Here's how the part is built. I have some questions about the finished solid (model axes, mm). A direction names the side the tool comes from. Coordinates: 2 decimals unless noted, no trailing zeros. Order: outer loops, then holes, each group sorted by start corner. A loop starts at its lowest first (then second) coordinate and runs counter-clockwise, first axis right, second up. Notation, with made-up numbers: (10.5, 8.25) - (60.5, 8.25) arc R31 cw to (60.5, 42.25) - close; hole circle Ø8 at (-36.75, -28). An arc over 180 degrees is marked (long way). Answer in a Markdown table with one row per item. Add a question column.
Item 1: Thinking about a two-plate mould opening in Z: for faces 1 (the flat face through (3.3, 0.1, -3.4)), 2 (the flat face through (1.03, 1.74, -0.99)), 3 (the cylindrical face through (18, -3, 0)), 4 (the conical face through (3.05, -0.07, -0.31)), which applies, +Z half, -Z half, draft (parallel to the pull), parting line (faces both ways), or undercut?
Item 2: If I drill on line 1 along Z through (x, y) = (26.5, 0); line 2 along Z through (x, y) = (1.5, -1); line 3 along X through (y, z) = (-2.75, -3.25), over which ranges is the centre line in solid material (lowest first)? Write a range as from..to.
Item 3: I want a section at A-A (x = 16). Please give me the cut outline in (y, z), plus the area to 3 significant figures.
Item 4: I want a section at B-B (y = 4.75). Please give me the cut outline in (x, z), plus the area to 3 significant figures.
Item 5: Will these pins go through, and if not, where does the flat tip stop? pin 1 Ø1 at (x, y) = (22.5, -2.5) entering from -Z; pin 2 Ø1.7 at (x, y) = (1, -0.5) entering from +Z; pin 3 Ø4 at (x, y) = (13.5, -2.5) entering from -Z; pin 4 Ø6 at (x, z) = (5, 0) entering from +Y.
Item 6: On a 3-axis mill with a long thin cutter (end or side, diameter ignored), from which of +Z, -Z, +X, -X, +Y, -Y can I reach the whole of each face in a straight line? I mean faces 5 (the flat face through (0, -2, -1)), 6 (the flat face through (1.03, -1.74, 0.99)). Say none if no direction works.
```python
from build123d import *

# Parameters (mm, degrees)
FILLET1_R   = 0.25
HEX_2_DEPTH = 2.08


with BuildPart() as part:
    # BodySke → BaseBody (revolve)
    with BuildSketch(Plane.XY):
        with BuildLine():
            Line((33.3, 0), (33.3, 2.4455))
            Line((33.3, 2.4455), (32.7455, 3))
            Line((32.7455, 3), (3.3, 3))
            Line((3.3, 3), (3.3, 5.25))
            Line((3.3, 5.25), (2.92, 5.25))
            ThreePointArc((2.92, 5.25), (1.224500646, 4.199464996), (0, 2.625))
            Line((0, 2.625), (0, 0))
            Line((0, 0), (33.3, 0))
        make_face()
    revolve(axis=Axis((0, 0, 0), (1, 0, 0)))

    # Fillet1
    fillet1_edges = [part.edges().sort_by_distance(p)[0] for p in [
        (3.3, -3, 0),
    ]]
    fillet(fillet1_edges, radius=FILLET1_R)

    # Sketch2 → PreBroach (revolve, cut)
    with BuildSketch(Plane.XY):
        Polygon((0, 2), (2.08, 2), (3.234700538, 0), (0, 0), align=None)
    revolve(axis=Axis((0, 0, 0), (1, 0, 0)), mode=Mode.SUBTRACT)

    # Sketch3 → Hex 2 (cut)
    with BuildSketch(Plane(origin=(0, 0, 0), x_dir=(0, 0, -1), z_dir=(1, 0, 0))):
        Polygon((-2, -1.154700538), (-2, 1.154700538), (0, 2.309401077), (2, 1.154700538), (2, -1.154700538), (0, -2.309401077), align=None)
    extrude(amount=HEX_2_DEPTH, mode=Mode.SUBTRACT)


solid = part.part
```
Values follow:
| question | item | result |
|---|---|---|
| 1 | face 1 | draft |
| 1 | face 2 | undercut |
| 1 | face 3 | parting line |
| 1 | face 4 | undercut |
| 2 | line 1 | z = -3..3 |
| 2 | line 2 | z = -4.32..-2, 2..4.32 |
| 2 | line 3 | x = 1.29..3.3 |
| 3 | outline | circle Ø6 at (0, 0) |
| 3 | area | 28.3 mm^2 |
| 4 | outline | (2.92, -2.24) - (3.3, -2.24) - (3.3, 2.24) - (2.92, 2.24) arc R3.05 ccw to start |
| 4 | area | 4.71 mm^2 |
| 5 | pin 1 | stops at z = -2.24 |
| 5 | pin 2 | stops at z = 4.67 |
| 5 | pin 3 | stops at z = -2.96 |
| 5 | pin 4 | stops at y = 5.25 |
| 6 | face 5 | +Z, -Z, -X, +Y, -Y |
| 6 | face 6 | -X |
